Source: CAD feature listing. Evaluate the final solid. Frame: model axes, mm. Face numbers are marked on the shaded views. A direction names the side the tool comes from. Round coordinates to 2 decimals unless told otherwise and drop trailing zeros. Loops run counter-clockwise (first coordinate to the right, second up) from the corner with the lowest first, then second, coordinate; pieces in that order, holes last. Notation, with made-up numbers: M 2.25,4 L 47.25,4 A24 cw 47.25,38 Z; hole C 49,44.5 d1. An arc over 180 degrees is marked long. One line per item, written item: value.
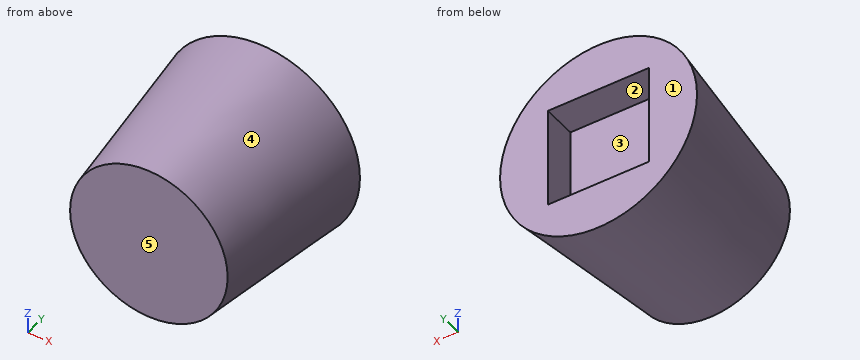
Autodesk Inventor part; units mm, degrees
ref_plane "YZ Plane" through (0, 0, 0) normal (1, 0, 0) x (0, 1, 0)
ref_plane "XZ Plane" through (0, 0, 0) normal (0, 1, 0) x (-1, 0, 0)
ref_plane "XY Plane" through (0, 0, 0) normal (0, 0, 1) x (1, 0, 0)
sketch "Эскиз1" plane through (0, 0, 0) normal (0, 0, 1) x (1, 0, 0)
  line L0 (0, 7.5) -> (0, -7.5)
  line L1 (0, 7.5) -> (8.75, 7.5)
  line L2 (8.75, 7.5) -> (7, -7.5)
  line L3 (7, -7.5) -> (0, -7.5)
  point P0 (0, 0)
  point P1 (0, 0)
  dimension "d0" = 15
  dimension "d1" = 17.5
  dimension "d2" = 14
revolve "Вращение1" add sketch "Эскиз1" angle 360 about axis through (0, 7.5, 0) along (0, -1, 0)
thread "Резьба1"
sketch "Эскиз3" plane through (0, 7.5, 0) normal (0, 1, 0) x (1, 0, 0)
  line L0 (-4.5, 4.5) -> (4.5, 4.5)
  line L1 (4.5, 4.5) -> (4.5, -4.5)
  line L2 (4.5, -4.5) -> (-4.5, -4.5)
  line L3 (-4.5, -4.5) -> (-4.5, 4.5)
  point P0 (0, 0)
  point P1 (-4.5, 0)
  point P2 (0, 4.5)
  dimension "d9" = 9
extrude "Выдавливание2" cut sketch "Эскиз3" against normal blind 3
properties part number "Пробка"
1. Ray query, line 1 (Y direction, x = 1, z = -3); line 2 (Z direction, x = 1.25, y = 6); line 3 (X direction, y = 4.75, z = -0.5). Return the intervals inside material, ascending. Write a range as [from, to].
Report:
line 1: y = [-7.5, 4.5]
line 2: z = [-8.48, -4.5], [4.5, 8.48]
line 3: x = [-8.41, -4.5], [4.5, 8.41]
2. Section query C-C (y = 5.25). Return the cut outline in (x, z) (1 decimal).
Report:
outline: C 0,0 d17; hole M -4.5,-4.5 L 4.5,-4.5 L 4.5,4.5 L -4.5,4.5 Z
3. Reachability of the marked faces 1 and 2 from +Z, -Z, +X, -X, +Y, -Y: full face, straight path, thin tool, end or side. Return the list, or none.
Report:
face 1: +Z, -Z, +X, -X, +Y
face 2: +Y
4. Section query B-B (x = 0). Return the cut outline in (y, z), and give its area (3 significant figures).
Report:
outline: M -7.5,-7 L 7.5,-8.75 L 7.5,-4.5 L 4.5,-4.5 L 4.5,4.5 L 7.5,4.5 L 7.5,8.75 L -7.5,7 Z
area: 209 mm2
5. Section query A-A (z = 0). Return the cut outline in (x, y).
Report:
outline: M -8.75,7.5 L -7,-7.5 L 7,-7.5 L 8.75,7.5 L 4.5,7.5 L 4.5,4.5 L -4.5,4.5 L -4.5,7.5 Z
6. Pin query (flat end, axial travel): pin 1 (4 mm diameter, centred on x = 1, y = 5, fed in from -Z); pin 2 (8 mm diameter, centred on x = 4.5, y = 2, fed in from -Z); pin 3 (8 mm diameter, centred on y = -0.5, z = 5, fed in from -X). Return the tip coordinate at first contact, or that it passes through.
Report:
pin 1: stops at z = -8.67
pin 2: stops at z = -8.29
pin 3: stops at x = -7.9
7. Section query D-D (y = 2.75). Return the cut outline in (x, z), and give its area (3 significant figures).
Report:
outline: C 0,0 d16.39
area: 211 mm2
8. Pull-direction query (X, two-part tool) for the marked faces 3, 4 and 5; classes: released by +X, released by -X, zero draft, split by the parting line, or undercut.
Report:
face 3: undercut
face 4: split by the parting line
face 5: zero draft
